```python
from build123d import *

# Parameters (mm, degrees)
F0_R      = 14
F1_DEPTH  = 11
F2_R      = 12
F3_DEPTH  = 32
F4_R      = 7.5
F4_R_2    = 4
F5_DEPTH  = 15
F6_R      = 7.5
F7_DEPTH  = 1
F8_R      = 6.15
F9_DEPTH  = 10
F10_R     = 1.5
F11_DEPTH = 25


with BuildPart() as f1:
    # F0 (on Front) → F1 (new body)
    with BuildSketch(Plane.XZ):
        Circle(F0_R)
    extrude(amount=F1_DEPTH)

    # F2 (on face) → F3 (join)
    with BuildSketch(Plane.XZ.offset(11)):
        Circle(F2_R)
    extrude(amount=F3_DEPTH)

    # F4 (on face) → F5 (join)
    with BuildSketch(Plane(origin=(0, 0, 0), x_dir=(-1, 0, 0), z_dir=(0, 1, 0))):
        Circle(F4_R)
        Circle(F4_R_2, mode=Mode.SUBTRACT)
    extrude(amount=F5_DEPTH)

    # F6 (on face) → F7 (join)
    with BuildSketch(Plane.XZ.offset(43)):
        Circle(F6_R)
    extrude(amount=F7_DEPTH)

    # F8 (on face) → F9 (join)
    with BuildSketch(Plane.XZ.offset(44)):
        Circle(F8_R)
    extrude(amount=F9_DEPTH)

    # F10 (on Right) → F11 (cut)
    with BuildSketch(Plane.YZ):
        with Locations((10, 0)):
            Circle(F10_R)
    extrude(amount=-F11_DEPTH, mode=Mode.SUBTRACT)


solid = f1.part
```
The model under review builds one solid part; all positions refer to its coordinate system, in mm. A direction names the side the tool comes from. Give positions to 0.01 mm unless a question says otherwise; leave off trailing zeros. Write each loop counter-clockwise with the first axis right and the second up, starting at its lowest first coordinate (ties: lowest second). Pieces come first, ordered by that corner, then holes. Notation, with made-up numbers: M 68.25,59.5 L 107.25,59.5 A24 ccw 107.25,97.5 Z; hole C 51,47.5 d7. An arc over 180 degrees is marked long. Answer in a Markdown table with one row per item.
Item 1: For line 1 along Z through (x, y) = (0, 4.75); line 2 along Y through (x, z) = (-4.6, 0); line 3 along Y through (x, z) = (1, -12.25), list the stretches that pass through material, from the lowest coordinate up.
Check sheet entries:
| item | result |
|---|---|
| line 1 | -7.5 to -4, 4 to 7.5 |
| line 2 | -54 to 8.5, 11.5 to 15 |
| line 3 | -11 to 0 |
Item 2: Draft analysis for pull direction Z (two halves, no side actions). For faces 1 (the face through (0, 0, 0)), 2 (the face through (12.932, -5.423, -5.362)), 3 (the face through (6, 0, -6)), state which applies: +Z half, -Z half, draft (parallel to the pull), parting line (faces both ways), or undercut.
Check sheet entries:
| item | result |
|---|---|
| face 1 | undercut |
| face 2 | parting line |
| face 3 | draft |
Item 3: Add section A-A on z = 0. Give the boundary of the cut face in (x, y).
Check sheet entries:
| item | result |
|---|---|
| outline | M -14,-11 L -12,-11 L -12,-43 L -7.5,-43 L -7.5,-44 L -6.15,-44 L -6.15,-54 L 6.15,-54 L 6.15,-44 L 7.5,-44 L 7.5,-43 L 12,-43 L 12,-11 L 14,-11 L 14,0 L 7.5,0 L 7.5,15 L 4,15 L 4,0 L -4,0 L -4,8.5 L -7.5,8.5 L -7.5,0 L -14,0 Z; M -7.5,11.5 L -4,11.5 L -4,15 L -7.5,15 Z |
Item 4: Add section B-B on x = 0. Give the boundary of the cut face in (y, z), plus the area to 3 significant figures.
Check sheet entries:
| item | result |
|---|---|
| outline | M -54,-6.15 L -44,-6.15 L -44,-7.5 L -43,-7.5 L -43,-12 L -11,-12 L -11,-14 L 0,-14 L 0,-7.5 L 15,-7.5 L 15,-4 L 0,-4 L 0,4 L 15,4 L 15,7.5 L 0,7.5 L 0,14 L -11,14 L -11,12 L -43,12 L -43,7.5 L -44,7.5 L -44,6.15 L -54,6.15 Z |
| area | 1,320 mm2 |
Item 5: Tool access review of faces 4 (the face through (-6, -44, 3)), 5 (the face through (-3, 15, -3)), 6 (the face through (7.493, 7.395, 0.33)), 7 (the face through (0, -54, 0)), 8 (the face through (-5.577, 9.805, 1.487)): name each direction out of +Z, -Z, +X, -X, +Y, -Y from which nothing blocks a thin tool from reaching the whole face with its end or side.
Check sheet entries:
| item | result |
|---|---|
| face 4 | -Y |
| face 5 | +Z, -Z, +X, -X, +Y |
| face 6 | +Y |
| face 7 | +Z, -Z, +X, -X, -Y |
| face 8 | -X |
Item 6: Add section C-C on z = -5.5. Give the boundary of the cut face in (x, y).
Check sheet entries:
| item | result |
|---|---|
| outline | M -12.87,-11 L -10.67,-11 L -10.67,-43 L -5.1,-43 L -5.1,-44 L -2.75,-44 L -2.75,-54 L 2.75,-54 L 2.75,-44 L 5.1,-44 L 5.1,-43 L 10.67,-43 L 10.67,-11 L 12.87,-11 L 12.87,0 L 5.1,0 L 5.1,15 L -5.1,15 L -5.1,0 L -12.87,0 Z |
Item 7: For P1, Ø12, axis at y = -12, z = -9, coming from the -X side; P2, Ø2, axis at x = -11, y = -10.5, coming from the +Z side; P3, Ø5, axis at x = 2, y = -35, coming from the -Z side, all flat-tipped, find the tip position at first contact; note any pin that passes through.
Check sheet entries:
| item | result |
|---|---|
| P1 | x = -13.66 |
| P2 | z = 9.8 |
| P3 | z = -12 |
Item 8: Add section D-D on y = -26. Give the boundary of the cut face in (x, z), plus the area to 3 significant figures.
Check sheet entries:
| item | result |
|---|---|
| outline | C 0,0 d24 |
| area | 452 mm2 |
